Can you work these out from the drawing? Everything is in mm from the part's minimum corner. A direction names the side the tool comes from. Give positions to 0.01 mm unless a question says otherwise; leave off trailing zeros. Loops run counter-clockwise (first coordinate to the right, second up) from the corner with the lowest first, then second, coordinate; pieces in that order, holes last. Notation, with made-up numbers: (-21, 82.5) - (33, 82.5) arc R28 ccw to (33, 113.5) - close; hole circle Ø4 at (28, 23). An arc over 180 degrees is marked (long way). Answer in a Markdown table with one row per item. Add a question column.
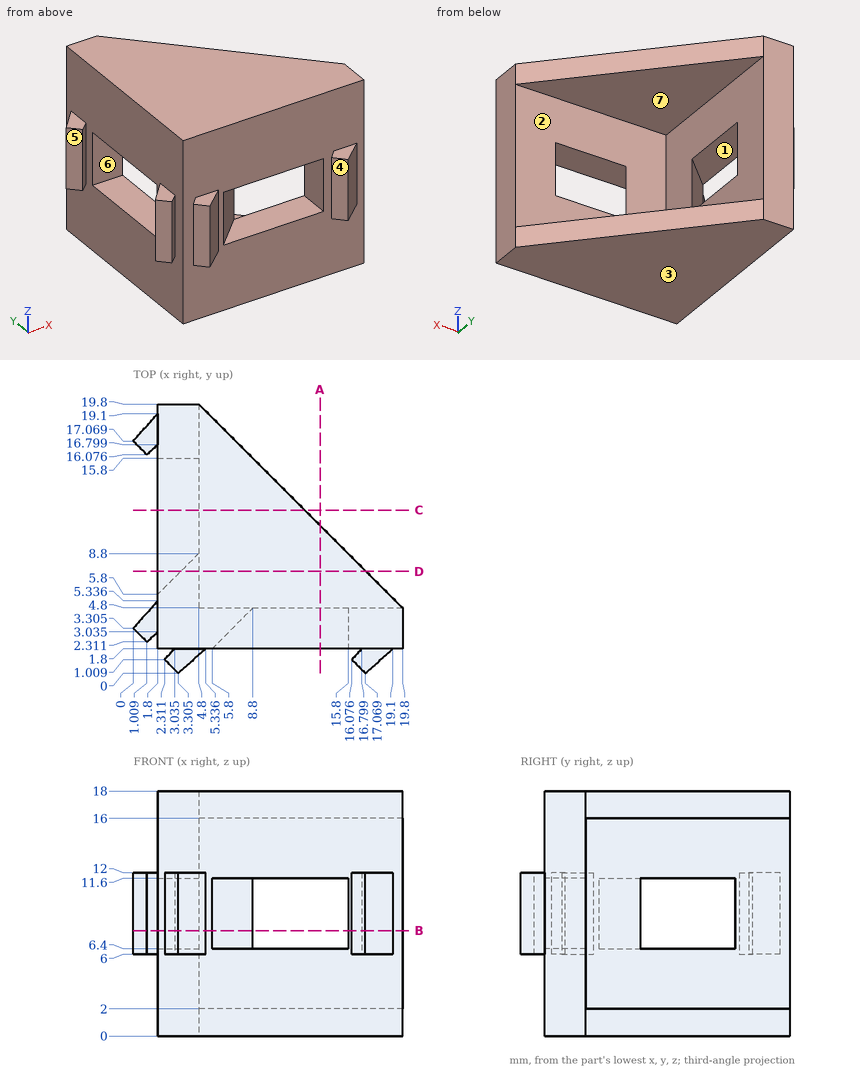
(1) Please list where these lines run through material, in increasing order: line 1 (Z direction, x = 4, y = 13.5); line 2 (Z direction, x = 19.25, y = 5); line 3 (X direction, y = 2.75, z = 13.5).
(2) I want a section at A-A on x = 13.75. Please give me the cut outline in (y, z).
(3) For pin 1 Ø1.4 at (x, y) = (17.5, 1) entering from +Z; pin 2 Ø0.9 at (x, y) = (1, 4) entering from -Z; pin 3 Ø9 at (x, z) = (8, 5) entering from -Y, each with a flat end and sliding along its axis, tell me the tip position at first contact or that it passes through.
(4) I want a section at C-C on y = 12. Please give me the cut outline in (x, z).
(5) I want a section at D-D on y = 7.5. Please give me the cut outline in (x, z).
(6) On a 3-axis mill with a long thin cutter (end or side, diameter ignored), from which of +Z, -Z, +X, -X, +Y, -Y can I reach the whole of each face in a straight line? I mean the marked faces 5, 6 and 7. Say none if no direction works.
(7) I want a section at B-B on z = 7.75. State how many separate pieces and enclosed holes the cut face has.
(8) We'd pull the mould along Y, two halves only. Please class the marked faces 1, 2, 3 and 4: pulls with the +Y half, pulls with the -Y half, needs draft (parallel to the pull), parting line crosses it, or undercut.
Reported:
| question | item | result |
|---|---|---|
| 1 | line 1 | 0 to 6.4, 11.6 to 18 |
| 1 | line 2 | 0 to 2, 16 to 18 |
| 1 | line 3 | 1.8 to 19.8 |
| 2 | outline | (1.8, 0) - (10.85, 0) - (10.85, 2) - (4.8, 2) - (4.8, 6.4) - (1.8, 6.4) - close; (1.8, 11.6) - (4.8, 11.6) - (4.8, 16) - (10.85, 16) - (10.85, 18) - (1.8, 18) - close |
| 3 | pin 1 | z = 12 |
| 3 | pin 2 | z = 6 |
| 3 | pin 3 | y = 0.27 |
| 4 | outline | (1.8, 0) - (12.6, 0) - (12.6, 2) - (4.8, 2) - (4.8, 6.4) - (1.8, 6.4) - close; (1.8, 11.6) - (4.8, 11.6) - (4.8, 16) - (12.6, 16) - (12.6, 18) - (1.8, 18) - close |
| 5 | outline | (1.8, 0) - (17.1, 0) - (17.1, 2) - (4.8, 2) - (4.8, 16) - (17.1, 16) - (17.1, 18) - (1.8, 18) - (1.8, 11.6) - (3.5, 11.6) - (3.5, 6.4) - (1.8, 6.4) - close |
| 6 | face 5 | +Z, -Z, -X |
| 6 | face 6 | +X, -X |
| 6 | face 7 | +X, +Y |
| 7 | separate pieces | 3 |
| 7 | enclosed holes | 0 |
| 8 | face 1 | undercut |
| 8 | face 2 | pulls with the +Y half |
| 8 | face 3 | needs draft |
| 8 | face 4 | pulls with the -Y half |
